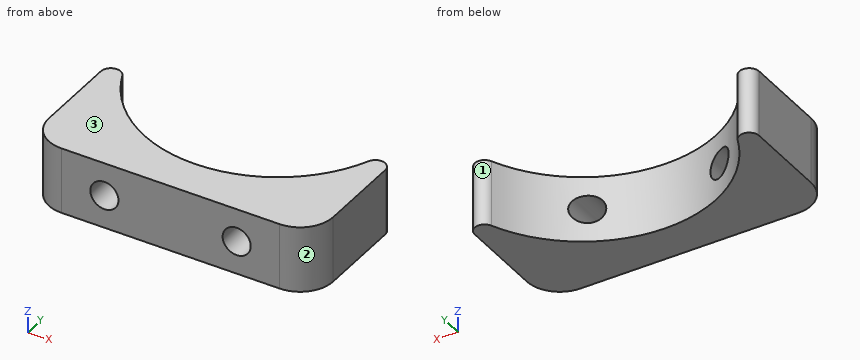
from build123d import *

# Parameters (mm, degrees)
BASE_EXTRUDE_DEPTH = 10
HOLE1_D            = 8.5
HOLE1_DEPTH        = 30
HOLE1_TIP          = 2.553657631


with BuildPart() as part:
    # Sketch1 → Base-Extrude (new body, symmetric)
    with BuildSketch(Plane.XY):
        with BuildLine():
            Line((43, -17.095320997), (43, -42.5))
            ThreePointArc((43, -42.5), (40.071067812, -49.571067812), (33, -52.5))
            Line((33, -52.5), (-33, -52.5))
            ThreePointArc((-33, -52.5), (-40.071067812, -49.571067812), (-43, -42.5))
            Line((-43, -42.5), (-43, -17.095320997))
            ThreePointArc((-43, -17.095320997), (-40.601721668, -14.156285265), (-37.24137931, -15.916333342))
            ThreePointArc((-37.24137931, -15.916333342), (0, -40.5), (37.24137931, -15.916333342))
            ThreePointArc((37.24137931, -15.916333342), (40.601721668, -14.156285265), (43, -17.095320997))
        make_face()
    extrude(amount=BASE_EXTRUDE_DEPTH, both=True)

    # Hole1
    with Locations(Plane.XZ.offset(52.5)):
        with Locations((-20, 0), (20, 0)):
            Hole(HOLE1_D / 2, depth=HOLE1_DEPTH)
            with Locations((0, 0, -(HOLE1_DEPTH + HOLE1_TIP / 2))):  # 118° drill point
                Cone(0, HOLE1_D / 2, HOLE1_TIP, mode=Mode.SUBTRACT)


solid = part.part
Geometry check sheet. Reference: the model listing, model coordinates, mm. Face numbers are marked on the shaded views. Coordinates: 2 decimals unless noted, no trailing zeros. Write each loop counter-clockwise with the first axis right and the second up, starting at its lowest first coordinate (ties: lowest second). Pieces come first, ordered by that corner, then holes. Notation, with made-up numbers: (22, -33.5) -> (76, -33.5) arc R14 ccw to (76, -19.5) -> close; hole circle Ø7 at (-4.5, 12.25). An arc over 180 degrees is marked (long way). One line per question, with ' | ' between items.
1. Thickness scan on probe 1 along Z at (x, y) = (20, -38); probe 2 along X at (y, z) = (-48.5, 0); probe 3 along X at (y, z) = (-37.25, 0). Record the ranges inside material, lowest first. Write a range as from..to.
Answers:
probe 1: z = -10..-4.25, 4.25..10 | probe 2: x = -41..-24.25, -15.75..15.75, 24.25..41 | probe 3: x = -43..-24.25, 24.25..43
2. Cross-section at B-B on y = -39. Record the cut outline in (x, z).
Answers:
outline: (-43, -10) -> (-10.92, -10) -> (-10.92, 10) -> (-43, 10) -> close; (10.92, -10) -> (43, -10) -> (43, 10) -> (10.92, 10) -> close; hole circle Ø8.5 at (-20, 0); hole circle Ø8.5 at (20, 0)
3. Depth check by flat-ended pin: pin 1 Ø4 at (x, z) = (-34, 2) entering from +Y; pin 2 Ø10 at (x, z) = (-20, 0) entering from -Y; pin 3 Ø10 at (x, z) = (-18, -5.5) entering from +Y. Enter the tip coordinate at first touch or a pass-through.
Answers:
pin 1: stops at y = -18.55 | pin 2: stops at y = -52.5 | pin 3: stops at y = -33.34
4. Cross-section at A-A on x = -20. Record the cut outline in (y, z), and give its area (3 significant figures).
Answers:
outline: (-52.5, -10) -> (-35.22, -10) -> (-35.22, -4.25) -> (-52.5, -4.25) -> close; (-52.5, 4.25) -> (-35.22, 4.25) -> (-35.22, 10) -> (-52.5, 10) -> close | area: 199 mm²
5. Draft check along X on the marked faces 1, 2 and 3. Enter one of: +X half, -X half, draft (parallel to the pull), parting line (faces both ways), or undercut.
Answers:
face 1: undercut | face 2: +X half | face 3: draft
6. Cross-section at C-C on z = 0. Record the cut outline in (x, y), and give its area (3 significant figures).
Answers:
outline: (-43, -42.5) arc R10 ccw to (-33, -52.5) -> (-24.25, -52.5) -> (-24.25, -32.44) arc R40.5 cw to (-37.24, -15.92) arc R3 ccw to (-43, -17.1) -> close; (-15.75, -52.5) -> (15.75, -52.5) -> (15.75, -37.31) arc R40.5 cw to (-15.75, -37.31) -> close; (24.25, -52.5) -> (33, -52.5) arc R10 ccw to (43, -42.5) -> (43, -17.1) arc R3 ccw to (37.24, -15.92) arc R40.5 cw to (24.25, -32.44) -> close | area: 1,500 mm²
7. Cross-section at D-D on y = -19. Record the cut outline in (x, z).
Answers:
outline: (-43, -10) -> (-35.77, -10) -> (-35.77, 10) -> (-43, 10) -> close; (35.77, -10) -> (43, -10) -> (43, 10) -> (35.77, 10) -> close
